from build123d import *

# Parameters (mm, degrees)
SKETCH1_W               = 40
SKETCH1_H               = 102
BOSS_EXTRUDE1_DEPTH     = 8.5
SKETCH2_W               = 35
SKETCH2_H               = 70
CUT_EXTRUDE1_DEPTH      = 3
SKETCH3_W               = 10.5
SKETCH3_H               = 10
CUT_EXTRUDE2_DEPTH      = 1.35
SKETCH4_W               = 12.5
SKETCH4_H               = 6
CUT_EXTRUDE3_DEPTH      = 3.1
SKETCH5_W               = 8.5
SKETCH5_H               = 17.5
PCB_PLACE_DEPTH         = 3.1
SKETCH6_W               = 8.5
SKETCH6_H               = 1.6
NICKEL_STRIP_HOLE_DEPTH = 66.369411807
CUT_EXTRUDE4_REACH      = 67.698
SKETCH7_W               = 8.5
SKETCH7_H               = 17.5
SKETCH8_W               = 8.5
SKETCH8_H               = 1.6
CUT_EXTRUDE5_DEPTH      = 10
SKETCH9_W               = 8.5
SKETCH9_H               = 102
NICKEL_STRIP_RAIL_DEPTH = 2.5
FILLET3_R               = 2.325
FILLET4_RADIUS          = 1.45
FILLET4_LENGTH          = 8.5
CUT_EXTRUDE6_REACH      = 106.289
SKETCH10_W              = 4.8
SKETCH10_H              = 4


with BuildPart() as part:
    # Sketch1 → Boss-Extrude1 (new body)
    with BuildSketch(Plane(origin=(0, 0, 0), x_dir=(1, 0, 0), z_dir=(0, 1, 0))):
        with Locations((0, 11)):
            Rectangle(SKETCH1_W, SKETCH1_H)
    extrude(amount=BOSS_EXTRUDE1_DEPTH)

    # Sketch2 → Cut-Extrude1 (cut)
    with BuildSketch(Plane(origin=(0, 8.5, 0), x_dir=(1, 0, 0), z_dir=(0, 1, 0))):
        with Locations((0, -2)):
            Rectangle(SKETCH2_W, SKETCH2_H)
    extrude(amount=-CUT_EXTRUDE1_DEPTH, mode=Mode.SUBTRACT)

    # Sketch3 → Cut-Extrude2 (cut)
    with BuildSketch(Plane(origin=(0, 8.5, 0), x_dir=(1, 0, 0), z_dir=(0, 1, 0))):
        with Locations((-6.65, 38)):
            Rectangle(SKETCH3_W, SKETCH3_H)
        with Locations((6.65, 38)):
            Rectangle(SKETCH3_W, SKETCH3_H)
    extrude(amount=-CUT_EXTRUDE2_DEPTH, mode=Mode.SUBTRACT)

    # Sketch4 → Cut-Extrude3 (cut)
    with BuildSketch(Plane(origin=(0, 8.5, 0), x_dir=(1, 0, 0), z_dir=(0, 1, 0))):
        with Locations((6.65, 40)):
            Rectangle(SKETCH4_W, SKETCH4_H)
    extrude(amount=-CUT_EXTRUDE3_DEPTH, mode=Mode.SUBTRACT)

    # Sketch5 → PCB place (cut)
    with BuildSketch(Plane(origin=(0, 8.5, 0), x_dir=(1, 0, 0), z_dir=(0, 1, 0))):
        with Locations((6.65, 51.75)):
            Rectangle(SKETCH5_W, SKETCH5_H)
    extrude(amount=-PCB_PLACE_DEPTH, mode=Mode.SUBTRACT)

    # Sketch6 → Nickel strip hole (cut, through all)
    with BuildSketch(Plane(origin=(0, 5.4, 0), x_dir=(1, 0, 0), z_dir=(0, 1, 0))):
        with Locations((6.65, 59.7)):
            Rectangle(SKETCH6_W, SKETCH6_H)
    extrude(amount=-NICKEL_STRIP_HOLE_DEPTH, mode=Mode.SUBTRACT)

    # Cut-Extrude4: up to this face of the body (flat: up to its plane)
    cut_extrude4_end = Plane(part.part.faces().sort_by_distance((6.65, 5.4, -47.042077088))[0])
    # Sketch7 → Cut-Extrude4 (cut, up to the picked face)
    with BuildSketch(Plane(origin=(0, 8.5, 0), x_dir=(1, 0, 0), z_dir=(0, 1, 0)), mode=Mode.PRIVATE) as cut_extrude4_sk1:
        with Locations((-6.65, 51.75)):
            Rectangle(SKETCH7_W, SKETCH7_H)
    cut_extrude4_tool1 = split(extrude(cut_extrude4_sk1.sketch, amount=-CUT_EXTRUDE4_REACH, mode=Mode.PRIVATE), bisect_by=cut_extrude4_end, keep=Keep.BOTH, mode=Mode.PRIVATE)
    add(cut_extrude4_tool1.solids().sort_by(Axis((-6.65, 8.5, -51.75), (0, -1, 0)))[0], mode=Mode.SUBTRACT)

    # Sketch8 → Cut-Extrude5 (cut)
    with BuildSketch(Plane(origin=(0, 5.4, 0), x_dir=(1, 0, 0), z_dir=(0, 1, 0))):
        with Locations((-6.65, 43.8)):
            Rectangle(SKETCH8_W, SKETCH8_H)
    extrude(amount=-CUT_EXTRUDE5_DEPTH, mode=Mode.SUBTRACT)

    # Sketch9 → Nickel strip rail (cut)
    with BuildSketch(Plane.XZ):
        with Locations((-6.65, -11)):
            Rectangle(SKETCH9_W, SKETCH9_H)
        with Locations((6.65, -11)):
            Rectangle(SKETCH9_W, SKETCH9_H)
    extrude(amount=-NICKEL_STRIP_RAIL_DEPTH, mode=Mode.SUBTRACT)

    # Fillet3
    # the kernel refuses this fillet: 2.325 mm, written as the material it takes off along each edge
    with BuildSketch(Plane(origin=(3.4125, 7.15, -43), x_dir=(0, 0, 1), z_dir=(-1, 0, 0))) as fillet3_piece_1_section:
        with BuildLine():
            CenterArc((FILLET3_R, -FILLET3_R), FILLET3_R, 90, 90)
            Line((0, -FILLET3_R), (0, 0))
            Line((0, 0), (FILLET3_R, 0))
        make_face()
    fillet3_piece_1 = extrude(amount=20.125, mode=Mode.PRIVATE)
    fillet3_piece_1 = split(fillet3_piece_1, bisect_by=Plane(origin=(-11.9, 7.15, -43), z_dir=(1, 0, 0)), keep=Keep.TOP, mode=Mode.PRIVATE)
    fillet3_piece_1 = split(fillet3_piece_1, bisect_by=Plane(origin=(-1.4, 7.15, -43), z_dir=(-1, 0, 0)), keep=Keep.TOP, mode=Mode.PRIVATE)
    add(fillet3_piece_1, mode=Mode.SUBTRACT)
    with BuildSketch(Plane(origin=(-10.9, 2.5, -43), x_dir=(0, 1, 0), z_dir=(1, 0, 0))) as fillet3_piece_2:
        with BuildLine():
            CenterArc((FILLET3_R, FILLET3_R), FILLET3_R, 180, 90)
            Line((0, FILLET3_R), (0, 0))
            Line((0, 0), (FILLET3_R, 0))
        make_face()
    extrude(amount=8.5, mode=Mode.SUBTRACT)

    # Fillet4: full round fillet: the end face becomes a half cylinder, R = half its width
    fillet4_face = Plane((6.65, 3.95, -58.9), x_dir=(-1, 0, 0), z_dir=(0, 0, -1))  # on the end face: x along it, z out of the body
    fillet4_slab = fillet4_face.offset(-FILLET4_RADIUS / 2) * Box(FILLET4_LENGTH, 2 * FILLET4_RADIUS, FILLET4_RADIUS, mode=Mode.PRIVATE)  # the body's end, R deep
    fillet4_round = Plane((6.65, 3.95, -57.45), x_dir=(0, 0, -1), z_dir=(-1, 0, 0)) * Cylinder(FILLET4_RADIUS, FILLET4_LENGTH, mode=Mode.PRIVATE)  # its axis R under the face
    add(fillet4_slab - fillet4_round, mode=Mode.SUBTRACT)

    # Cut-Extrude6: up to this face of the body (flat: up to its plane)
    cut_extrude6_end = Plane(part.part.faces().sort_by_distance((0, 4.678571429, -62))[0])
    # Sketch10 → Cut-Extrude6 (cut, up to the picked face)
    with BuildSketch(Plane.XY.offset(40), mode=Mode.PRIVATE) as cut_extrude6_sk1:
        with Locations((0, 2)):
            Rectangle(SKETCH10_W, SKETCH10_H)
    cut_extrude6_tool1 = split(extrude(cut_extrude6_sk1.sketch, amount=-CUT_EXTRUDE6_REACH, mode=Mode.PRIVATE), bisect_by=cut_extrude6_end, keep=Keep.BOTH, mode=Mode.PRIVATE)
    add(cut_extrude6_tool1.solids().sort_by(Axis((0, 2, 40), (0, 0, -1)))[0], mode=Mode.SUBTRACT)


solid = part.part
Read the model definition and answer for the solid it produces. Units are mm, in the model's axes. A direction names the side the tool comes from. Coordinates: 2 decimals unless noted, no trailing zeros. Loops run counter-clockwise (first coordinate to the right, second up) from the corner with the lowest first, then second, coordinate; pieces in that order, holes last.
Q1. Consider probe 1 along Z at (x, y) = (8, 6.25); probe 2 along X at (y, z) = (5.5, -46); probe 3 along X at (y, z) = (1.25, -12). Determine where each line is inside the solid, lowest interval first.
Q2. Which of the six approach directions +Z, -Z, +X, -X, +Y, -Y give full straight-line access (tool end or side, diameter ignored) to faces 1 (the face through (17.5, 7, 2)), 2 (the face through (7, 2.5, -8)), 3 (the face through (0, 5, 40))?
Q3. The part is cut by section A-A on z = -4. Write down the section's boundary in (x, y), and give its area (3 significant figures).
Q4. The part is cut by section B-B on x = 14. Write down the section's boundary in (y, z), and give its area (3 significant figures).
Q5. Each of these flat-tipped pins is pushed along its axis until it touches: pin 1 Ø1 at (x, z) = (-9.5, -28) entering from +Y; pin 2 Ø7 at (x, z) = (-5.5, -53.5) entering from -Y; pin 3 Ø3 at (x, z) = (4.5, -35.5) entering from +Y. Where does it stop, or does it pass through?
Results below:
1. probe 1: z = -62 to -60.5, -37 to -33, 37 to 40
1. probe 2: x = -20 to -10.9, -2.4 to 2.4, 10.9 to 20
1. probe 3: x = -20 to -10.9, 10.9 to 20
2. face 1: +Y
2. face 2: +Z, -Z, -Y
2. face 3: +Z, +X, -X, +Y, -Y
3. outline: (-20, 0) - (-10.9, 0) - (-10.9, 2.5) - (-2.4, 2.5) - (-2.4, 4) - (2.4, 4) - (2.4, 2.5) - (10.9, 2.5) - (10.9, 0) - (20, 0) - (20, 8.5) - (17.5, 8.5) - (17.5, 5.5) - (-17.5, 5.5) - (-17.5, 8.5) - (-20, 8.5) - close
3. area: 173 mm2
4. outline: (0, -62) - (8.5, -62) - (8.5, -33) - (5.5, -33) - (5.5, 37) - (8.5, 37) - (8.5, 40) - (0, 40) - close
4. area: 657 mm2
5. pin 1: stops at y = 5.5
5. pin 2: stops at y = 2.5
5. pin 3: stops at y = 7.15
